The drawing under review shows one solid part. Ordinate dimensions are in mm from its lowest x, y, z. A direction names the side the tool comes from. Coordinates: 2 decimals unless noted, no trailing zeros. Write each loop counter-clockwise with the first axis right and the second up, starting at its lowest first coordinate (ties: lowest second). Pieces come first, ordered by that corner, then holes. Notation, with made-up numbers: (79, 68.5) - (109, 68.5) arc R22 cw to (109, 100.5) - close; hole circle Ø1 at (32, 15.25). An arc over 180 degrees is marked (long way). Use a Markdown table: item, result.
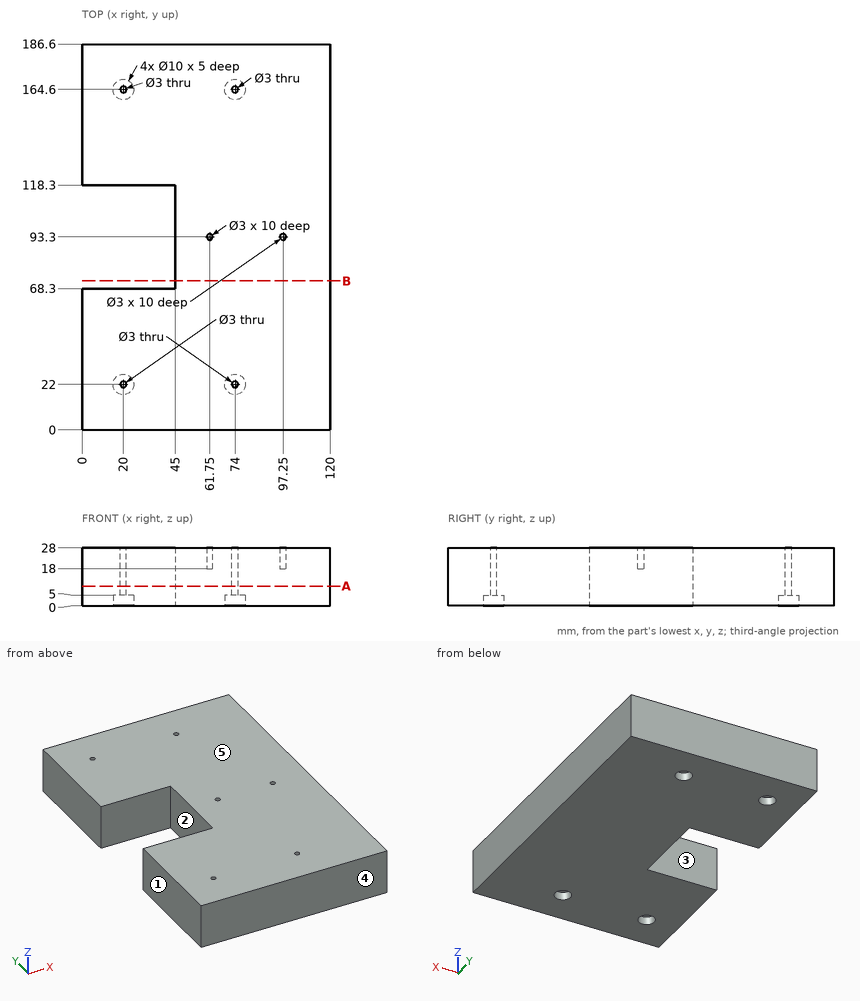
(1) Take a section at A-A on z = 9.5. Write out the cut boundary in (x, y).
Determined:
| item | result |
|---|---|
| outline | (0, 0) - (120, 0) - (120, 186.6) - (0, 186.6) - (0, 118.3) - (45, 118.3) - (45, 68.3) - (0, 68.3) - close; hole circle Ø3 at (20, 22); hole circle Ø3 at (20, 164.6); hole circle Ø3 at (74, 22); hole circle Ø3 at (74, 164.6) |
(2) For pin 1 (12 mm diameter, centred on y = 96, z = 24.5, fed in from -X); pin 2 (2.5 mm diameter, centred on x = 61.75, y = 93.3, fed in from +Z); pin 3 (5 mm diameter, centred on x = 75, y = 20, fed in from -Z), all flat-tipped, find the tip position at first contact; note any pin that passes through.
Determined:
| item | result |
|---|---|
| pin 1 | x = 45 |
| pin 2 | z = 18 |
| pin 3 | z = 5 |
(3) For L1, parallel to Y at x = 20, z = 2.1; L2, parallel to X at y = 93.3, z = 25.25; L3, parallel to Y at x = 20, z = 19.5, list the stretches that pass through material, from the lowest coordinate up. Write a range as from..to.
Determined:
| item | result |
|---|---|
| L1 | 0..17, 27..68.3, 118.3..159.6, 169.6..186.6 |
| L2 | 45..60.25, 63.25..95.75, 98.75..120 |
| L3 | 0..20.5, 23.5..68.3, 118.3..163.1, 166.1..186.6 |
(4) Machinability: for the marked faces 1 and 2, which of the approach directions +Z, -Z, +X, -X, +Y, -Y give a long, thin tool a straight path to every point of the face, cutting with its end or side? Answer none if there is none.
Determined:
| item | result |
|---|---|
| face 1 | +Z, -Z, -X, +Y, -Y |
| face 2 | +Z, -Z, -X |
(5) Draft analysis for pull direction Y (two halves, no side actions). For the marked faces 3, 4 and 5, state which applies: +Y half, -Y half, draft (parallel to the pull), parting line (faces both ways), or undercut.
Determined:
| item | result |
|---|---|
| face 3 | undercut |
| face 4 | -Y half |
| face 5 | draft |
(6) Take a section at B-B on y = 72. Write out the cut boundary in (x, z), and give its area (3 significant figures).
Determined:
| item | result |
|---|---|
| outline | (45, 0) - (120, 0) - (120, 28) - (45, 28) - close |
| area | 2,100 mm2 |
